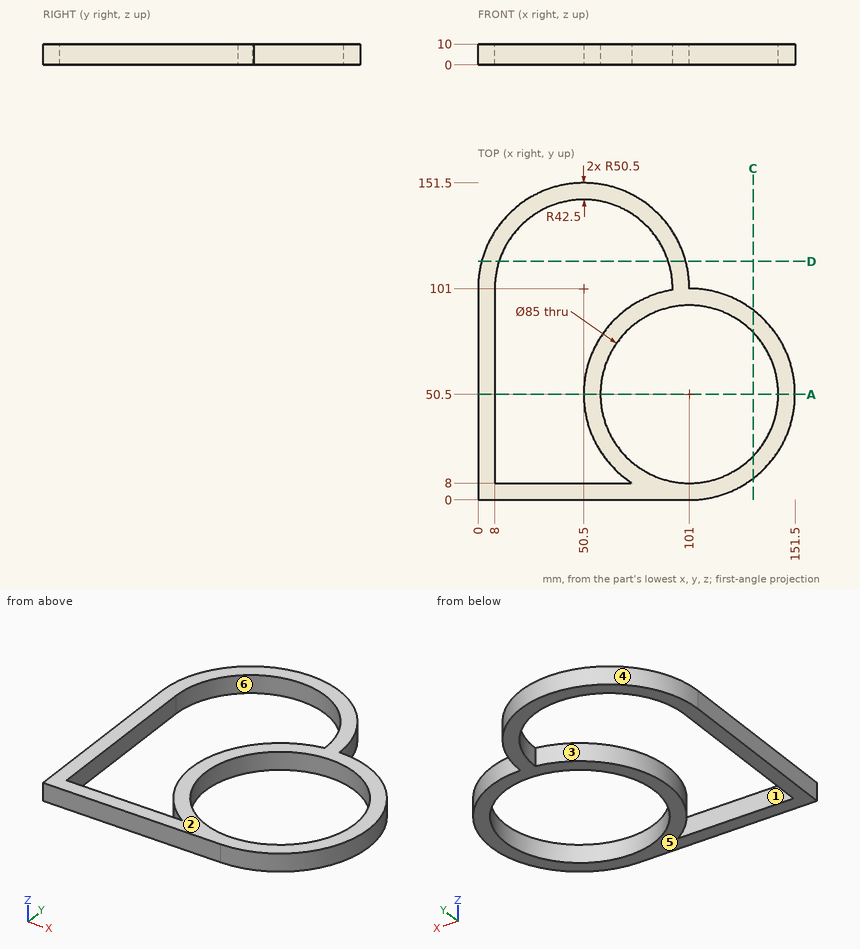
Geometry check sheet. Reference: drawing and pictorial views, mm from the part's lowest x, y, z. A direction names the side the tool comes from. Round coordinates to 2 decimals unless told otherwise and drop trailing zeros. Loops run counter-clockwise (first coordinate to the right, second up) from the corner with the lowest first, then second, coordinate; pieces in that order, holes last. Notation, with made-up numbers: M 17,-16 L 76,-16 A20 cw 76,12 Z; hole C 72,39.25 d5. An arc over 180 degrees is marked long. Return JSON: item names as keys, results as strings. Group by question number.
(1) Section check A-A, the plane y = 50.5. Enter the section's corners in (x, z).
(2) Section check D-D, the plane y = 114. Enter the section's corners in (x, z), and give its area (3 significant figures).
(3) Section check C-C, the plane x = 131.5. Enter the section's corners in (y, z).
(4) Set-up check for the marked faces 1 and 2: record each of +Z, -Z, +X, -X, +Y, -Y from which the full face is reachable in a straight line by a thin tool's end or side.
(5) Mould release check, pull along Y, two halves, no side actions. Record for the marked faces 3, 4, 5 and 6: pulls with the +Y half, pulls with the -Y half, needs draft (parallel to the pull), parting line crosses it, or undercut.
(6) Go/stop test with flat-tipped pins: pin 1 (3 mm diameter, centred on x = 116.5, z = 3, fed in from -Y); pin 2 (3 mm diameter, centred on y = 72, z = 4, fed in from +X). Record where each tip stops, or that it passes through.
(7) Scan lines: line 1 along Y through (x, z) = (57, 7.5); line 2 along Y through (x, z) = (68.5, 7.75); line 3 along Y through (x, z) = (54.5, 4.5). Record each from-to range of solid material in increasing order. Write a range as [from, to].
Data:
{
 "1": {"outline": "M 0,0 L 8,0 L 8,10 L 0,10 Z; M 50.5,0 L 58.5,0 L 58.5,10 L 50.5,10 Z; M 143.5,0 L 151.5,0 L 151.5,10 L 143.5,10 Z"},
 "2": {"outline": "M 1.7,0 L 10.04,0 L 10.04,10 L 1.7,10 Z; M 90.96,0 L 99.3,0 L 99.3,10 L 90.96,10 Z", "area": "167 mm²"},
 "3": {"outline": "M 10.25,0 L 20.9,0 L 20.9,10 L 10.25,10 Z; M 80.1,0 L 90.75,0 L 90.75,10 L 80.1,10 Z"},
 "4": {"face 1": "+Z, -Z", "face 2": "+Z, +X, -X, +Y, -Y"},
 "5": {"face 3": "undercut", "face 4": "pulls with the +Y half", "face 5": "needs draft", "face 6": "undercut"},
 "6": {"pin 1": "y = 1.98", "pin 2": "x = 147.37"},
 "7": {"line 1": "[0, 8], [25.72, 75.28], [143, 151.08]", "line 2": "[0, 8], [11.85, 23.11], [77.89, 89.15], [139.5, 148.18]", "line 3": "[0, 8], [30.8, 70.2], [143.31, 151.34]"}
}
